```python
from build123d import *

# Parameters (mm, degrees)
BOSS_EXTRUDE1_DEPTH = 3
SKETCH3_R           = 4
CUT_EXTRUDE1_DEPTH  = 3
FILLET2_R           = 3
FILLET3_R           = 3
FILLET4_R           = 3
FILLET5_R           = 3


with BuildPart() as part:
    # Sketch2 → Boss-Extrude1 (new body)
    with BuildSketch(Plane.XY):
        with BuildLine():
            Line((0, 10), (90, 10))
            Line((90, 10), (185.282890453, 26.800944387))
            ThreePointArc((185.282890453, 26.800944387), (212.182976557, 20.837338873), (226.987303957, -2.400800326))
            Line((226.987303957, -2.400800326), (189.399599126, 11.280005407))
            Line((189.399599126, 11.280005407), (177.770914253, -20.669543699))
            Line((177.770914253, -20.669543699), (216.366079007, -34.717034857))
            ThreePointArc((216.366079007, -34.717034857), (198.899834433, -43.890576734), (179.221499689, -42.48106907))
            Line((179.221499689, -42.48106907), (89.98049586, -10))
            Line((89.98049586, -10), (0, -10))
            ThreePointArc((0, -10), (-10, 0), (0, 10))
        make_face()
    extrude(amount=BOSS_EXTRUDE1_DEPTH)

    # Sketch3 → Cut-Extrude1 (cut)
    with BuildSketch(Plane.XY.offset(3)):
        Circle(SKETCH3_R)
        Polygon((147, -16.85066389), (158, -10.499810929), (158, 2.201894993), (147, 8.552747954), (136, 2.201894993), (136, -10.499810929), align=None)
    extrude(amount=-CUT_EXTRUDE1_DEPTH, mode=Mode.SUBTRACT)

    # Fillet2
    fillet2_edges = [part.edges().sort_by_distance(p)[0] for p in [
        (216.366079007, -34.717034857, 1.5),
    ]]
    fillet(fillet2_edges, radius=FILLET2_R)

    # Fillet3
    fillet3_edges = [part.edges().sort_by_distance(p)[0] for p in [
        (226.987303957, -2.400800326, 1.5),
    ]]
    fillet(fillet3_edges, radius=FILLET3_R)

    # Fillet4
    fillet4_edges = [part.edges().sort_by_distance(p)[0] for p in [
        (177.770914253, -20.669543699, 1.5),
    ]]
    fillet(fillet4_edges, radius=FILLET4_R)

    # Fillet5
    fillet5_edges = [part.edges().sort_by_distance(p)[0] for p in [
        (189.399599126, 11.280005407, 1.5),
    ]]
    fillet(fillet5_edges, radius=FILLET5_R)


solid = part.part
```
Part model, mm, in its own coordinate system. A direction names the side the tool comes from. Coordinates: 2 decimals unless noted, no trailing zeros. Write each loop counter-clockwise with the first axis right and the second up, starting at its lowest first coordinate (ties: lowest second). Pieces come first, ordered by that corner, then holes.
Item 1: Slice it at A-A (z = 0.6). Write the cut outline in (x, y) (1 decimal), and give its area (3 significant figures).
Item 2: Which spindle directions (+Z, -Z, +X, -X, +Y, -Y) get a long thin tool onto all of the face, cutting with end or side? Do faces 1 (the face through (109, 0, 3)), 2 (the face through (141.42, -13.63, 1.52)). Say none if no direction does.
Item 3: Pin check, flat tips, straight feed: pin 1 (1.5 mm diameter, centred on x = 48, z = 2, fed in from +Y); pin 2 (0.9 mm diameter, centred on y = -3, z = 1.5, fed in from +X); pin 3 (1 mm diameter, centred on x = 179, z = 1, fed in from -Y). Stop position of each tip, or through.
Item 4: Slice it at B-B (x = 145). Write the cut outline in (y, z).
Item 5: Mould opens along X. For faces 3 (the face through (196.42, -44.32, 1.48)), 4 (the face through (109, 0, 0)), 5 (the face through (195.79, -27.23, 1.48)), 6 (the face through (152.42, -13.72, 1.52)) say: released by +X, released by -X, zero draft, split by the parting line, or undercut.
Item 6: Slice it at C-C (x = 21.5). Write the cut outline in (y, z), and give its area (3 significant figures).
Item 7: Probe line 1 (Y direction, x = 0, z = 0.65); line 2 (Y direction, x = 26, z = 0.7); line 3 (X direction, y = -8, z = 2.15). List the from-to ranges inside material, lowest first.
Item 8: Slice it at D-D (y = -26). Write the cut outline in (x, z).
Results found:
1. outline: (0, -10) - (90, -10) - (179.2, -42.5) arc R36 ccw to (212.1, -38.2) arc R3 ccw to (211.4, -32.9) - (180.6, -21.7) arc R3 cw to (178.8, -17.9) - (188.4, 8.5) arc R3 cw to (192.2, 10.3) - (221.6, -0.4) arc R3 ccw to (225.5, 3.4) arc R36 ccw to (185.3, 26.8) - (90, 10) - (0, 10) arc R10 ccw to start; hole circle Ø8 at (0, 0); hole (136, -10.5) - (147, -16.9) - (158, -10.5) - (158, 2.2) - (147, 8.6) - (136, 2.2) - close
1. area: 6,840 mm2
2. face 1: +Z, +X, -X, +Y, -Y
2. face 2: +Z, -Z
3. pin 1: stops at y = 10
3. pin 2: stops at x = 184.37
3. pin 3: stops at y = -42.58
4. outline: (-30.03, 0) - (-15.7, 0) - (-15.7, 3) - (-30.03, 3) - close; (7.4, 0) - (19.7, 0) - (19.7, 3) - (7.4, 3) - close
5. face 3: split by the parting line
5. face 4: zero draft
5. face 5: released by +X
5. face 6: undercut
6. outline: (-10, 0) - (10, 0) - (10, 3) - (-10, 3) - close
6. area: 60.0 mm2
7. line 1: y = -10 to -4, 4 to 10
7. line 2: y = -10 to 10
7. line 3: x = -6 to 136, 158 to 182.38
8. outline: (133.94, 0) - (192.42, 0) - (192.42, 3) - (133.94, 3) - close
